The model under review builds one solid part; all positions refer to its coordinate system, in mm. A direction names the side the tool comes from. Give positions to 0.01 mm unless a question says otherwise; leave off trailing zeros. Loops run counter-clockwise (first coordinate to the right, second up) from the corner with the lowest first, then second, coordinate; pieces in that order, holes last. Notation, with made-up numbers: (86, 9.5) -> (94, 9.5) arc R19 ccw to (94, 38.5) -> close; hole circle Ø4 at (59, 50.5). An arc over 180 degrees is marked (long way). Write each question's results on one line, items separated by ' | '. Start each with the question number.
Q1. We need section C-C (z = 6.35). Give the number of separate pieces and of enclosed holes in the cut face, plus the area to 3 significant figures.
Q2. We need section D-D (x = -21.59). Write out the cut boundary in (y, z).
Q3. Wall thickness on L1, parallel to X at y = 11, z = 12.25; L2, parallel to Y at x = 21.5, z = 1.75; L3, parallel to Z at x = -21.59, y = -1: over which ranges is each line inside the solid? List them lowest first. Write a range as [from, to].
Q4. Machinability: for faces 1 (the face through (-18, 0, 6)), 2 (the face through (15.99, 22.88, 7.11)), 3 (the face through (24.13, 20, 6)), 4 (the face through (7.62, 7, 6)), which of the approach directions +Z, -Z, +X, -X, +Y, -Y give a long, thin tool a straight path to every point of the face, cutting with its end or side? Answer none if there is none.
Q5. Insertion check: pin 1 Ø2 at (x, z) = (-5.5, 9.5) entering from +Y; pin 2 Ø3 at (y, z) = (20, 9) entering from -X; pin 3 Ø1 at (y, z) = (9, 8) entering from -X. Each pin has a flat end and moves straight along its axis. Give the tip position at first contact, or say it passes through.
Q6. We need section B-B (y = 8). Write out the cut boundary in (x, z).
Q7. We need section A-A (x = 13.5). Write out the cut boundary in (y, z).
Q8. Mouldability with a two-part tool opening along Y and no side actions: class faces 5 (the face through (5.08, 8, 6)), 6 (the face through (2.54, 13, 6)), 7 (the face through (0.91, 23.18, 6.44)), 8 (the face through (2, 11, 12.7)) as released by +Y, released by -Y, zero draft, split by the parting line, or undercut.
from build123d import *

# Parameters (mm, degrees)
F1_DEPTH  = 12.7
F2_R      = 3.175
F3_W      = 33.02
F3_H      = 12.7
F4_DEPTH  = 2.54
F5_R      = 5.08
F6_R      = 2.4892
F7_DEPTH  = 2.54
F8_R      = 2.54
F9_DEPTH  = 2.54
F10_R     = 2.54
F11_DEPTH = 2.54


with BuildPart() as f1:
    # F0 (on Top) → F1 (new body)
    with BuildSketch(Plane.XY):
        Polygon((0, 24.13), (0, -2.1948770154), (0, -2.54), (7.62, -2.54), (7.62, 16.51), (26.67, 16.51), (26.67, 24.13), align=None)
        Polygon((5.08, 0), (2.54, 0), (2.54, 21.59), (5.08, 21.59), (24.13, 21.59), (24.13, 19.05), (5.08, 19.05), align=None, mode=Mode.SUBTRACT)
    extrude(amount=F1_DEPTH)

    # F2
    f2_edges = [f1.edges().sort_by_distance(p)[0] for p in [
        (26.67, 24.13, 6.35),
        (26.67, 16.51, 6.35),
        (5.08, 19.05, 6.35),
        (0, 24.13, 6.35),
        (7.62, -2.54, 6.35),
        (0, -2.54, 6.35),
        (7.62, 16.51, 6.35),
    ]]
    fillet(f2_edges, radius=F2_R)

    # F3 (on face) → F4 (join)
    with BuildSketch(Plane.XZ.offset(2.54)):
        with Locations((-13.335, 6.35)):
            Rectangle(F3_W, F3_H)
    extrude(amount=-F4_DEPTH)

    # F5
    f5_edges = [f1.edges().sort_by_distance(p)[0] for p in [
        (0.064148, 0, 6.35),
    ]]
    fillet(f5_edges, radius=F5_R)

    # F6 (on face) → F7 (cut, through all)
    with BuildSketch(Plane.XZ.offset(2.54)):
        with Locations((-21.59, 6.35)):
            Circle(F6_R)
    extrude(amount=-F7_DEPTH, mode=Mode.SUBTRACT)

    # F8 (on face) → F9 (cut, through all)
    with BuildSketch(Plane(origin=(0, 24.13, 0), x_dir=(-1, 0, 0), z_dir=(0, 1, 0))):
        with Locations((-18.415, 6.35)):
            Circle(F8_R)
    extrude(amount=-F9_DEPTH, mode=Mode.SUBTRACT)

    # F10 (on face) → F11 (cut, through all)
    with BuildSketch(Plane(origin=(0, 0, 0), x_dir=(0, -1, 0), z_dir=(-1, 0, 0))):
        with Locations((-9.525, 6.35)):
            Circle(F10_R)
    extrude(amount=-F11_DEPTH, mode=Mode.SUBTRACT)


solid = f1.part
Output:
1) separate pieces: 3 | enclosed holes: 0 | area: 279 mm2
2) outline: (-2.54, 0) -> (0, 0) -> (0, 3.86) -> (-2.54, 3.86) -> close; (-2.54, 8.84) -> (0, 8.84) -> (0, 12.7) -> (-2.54, 12.7) -> close
3) L1: [0, 2.54], [5.08, 7.62] | L2: [16.51, 19.05], [21.59, 24.13] | L3: [0, 3.86], [8.84, 12.7]
4) face 1: +Z, -Z, -X, +Y | face 2: +Y | face 3: +Z, -Z | face 4: +Z, -Z, +X, -Y
5) pin 1: y = 0.03 | pin 2: x = 0 | pin 3: x = 5.08
6) outline: (0, 0) -> (2.54, 0) -> (2.54, 4.32) -> (0, 4.32) -> close; (0, 8.38) -> (2.54, 8.38) -> (2.54, 12.7) -> (0, 12.7) -> close; (5.08, 0) -> (7.62, 0) -> (7.62, 12.7) -> (5.08, 12.7) -> close
7) outline: (16.51, 0) -> (19.05, 0) -> (19.05, 12.7) -> (16.51, 12.7) -> close; (21.59, 0) -> (24.13, 0) -> (24.13, 12.7) -> (21.59, 12.7) -> close
8) face 5: undercut | face 6: undercut | face 7: released by +Y | face 8: zero draft
